Geometry: final body of the model. Coordinates: model frame, mm. Face numbers are marked on the shaded views. A direction names the side the tool comes from. Give positions to 0.01 mm unless a question says otherwise; leave off trailing zeros. Write each loop counter-clockwise with the first axis right and the second up, starting at its lowest first coordinate (ties: lowest second). Pieces come first, ordered by that corner, then holes. Notation, with made-up numbers: M 41,60 L 76,60 A27 ccw 76,91 Z; hole C 33,45.25 d2. An arc over 180 degrees is marked long. Use a Markdown table: item, result. Add a question column.
1) Section A-A on y = 5. Return the cut outline in (x, z), then the cut area to 3 significant figures.
2) Section B-B on x = -9.5. Return the cut outline in (y, z).
3) Set-up query: the marked faces 5, 6 and 7. Return all of +Z, -Z, +X, -X, +Y, -Y with unobstructed straight access to the full face (end or side cutting, diameter ignored); none if empty.
4) Line query: line 1 (Z direction, x = 17.5, y = 14); line 2 (Z direction, x = -27, y = 16); line 3 (Z direction, x = 2, y = 9). Output: solid intervals per line, ascending.
5) Pin query (flat end, axial travel): pin 1 (5 mm diameter, centred on x = 16.5, y = 1, fed in from +Z); pin 2 (1 mm diameter, centred on y = 5, z = 18.5, fed in from +X); pin 3 (1.5 mm diameter, centred on x = 5.5, z = 21, fed in from +Y); pin 4 (8 mm diameter, centred on x = -9.5, y = 12.5, fed in from +Z). Return the tip coordinate at first contact, or that it passes through.
6) Draft query along X for the marked faces 1, 2, 3 and 4. Return one class per face: +X half, -X half, draft (parallel to the pull), parting line (faces both ways), or undercut.
7) Section C-C on y = -6.5. Return the cut outline in (x, z), then the cut area to 3 significant figures.
8) Section D-D on z = 21.5. Return the cut outline in (x, y).
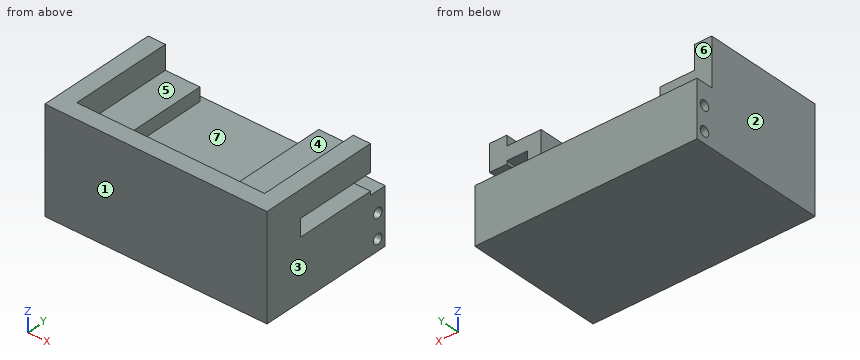
```python
from build123d import *

# Parameters (mm, degrees)
ESQUISSE1_W             = 54.5
ESQUISSE1_H             = 30
BOSS_EXTRU_8_DEPTH      = 5
ESQUISSE7_W             = 30
ESQUISSE7_H             = 30
BOSS_EXTRU_9_DEPTH      = 5
ESQUISSE8_W             = 30
ESQUISSE8_H             = 30
BOSS_EXTRU_10_DEPTH     = 5
ESQUISSE9_W             = 64.5
ESQUISSE9_H             = 30
BOSS_EXTRU_11_DEPTH     = 5
ESQUISSE10_W            = 5
ESQUISSE10_H            = 30
BOSS_EXTRU_12_DEPTH     = 55
ESQUISSE11_W            = 64.5
ESQUISSE11_H            = 16.16204781
BOSS_EXTRU_13_DEPTH     = 5
ESQUISSE13_W            = 3.918976095
ESQUISSE13_H            = 30
BOSS_EXTRU_14_DEPTH     = 10
ESQUISSE16_W            = 3.9189761
ESQUISSE16_H            = 30
BOSS_EXTRU_15_DEPTH     = 10
ESQUISSE17_W            = 3.9189761
ESQUISSE17_H            = 30
BOSS_EXTRU_16_DEPTH     = 4
ESQUISSE20_W            = 5
ESQUISSE20_H            = 23.625106292
ENL_V_MAT_EXTRU_2_DEPTH = 7
ESQUISSE21_R            = 1.45
ENL_V_MAT_EXTRU_3_DEPTH = 7
ENL_V_START             = -7
ESQUISSE22_R            = 1.45
ENL_V_MAT_EXTRU_4_DEPTH = 7


with BuildPart() as part:
    # Esquisse1 → Boss.-Extru.8 (new body)
    with BuildSketch(Plane.XY):
        with Locations((-8.335450003, 5.161172161)):
            Rectangle(ESQUISSE1_W, ESQUISSE1_H)
    extrude(amount=BOSS_EXTRU_8_DEPTH)

    # Esquisse7 → Boss.-Extru.9 (add)
    with BuildSketch(Plane.ZY.offset(35.585450003)):
        with Locations((15, 5.161172161)):
            Rectangle(ESQUISSE7_W, ESQUISSE7_H)
    extrude(amount=BOSS_EXTRU_9_DEPTH)

    # Esquisse8 → Boss.-Extru.10 (add)
    with BuildSketch(Plane(origin=(18.914549997, 0, 0), x_dir=(0, 0, -1), z_dir=(1, 0, 0))):
        with Locations((-15, 5.161172161)):
            Rectangle(ESQUISSE8_W, ESQUISSE8_H)
    extrude(amount=BOSS_EXTRU_10_DEPTH)

    # Esquisse9 → Boss.-Extru.11 (add)
    with BuildSketch(Plane.XZ.offset(9.838827839)):
        with Locations((-8.335450003, 15)):
            Rectangle(ESQUISSE9_W, ESQUISSE9_H)
    extrude(amount=BOSS_EXTRU_11_DEPTH)

    # Esquisse10 → Boss.-Extru.12 (add)
    with BuildSketch(Plane(origin=(-35.585450003, 0, 0), x_dir=(0, 0, -1), z_dir=(1, 0, 0))):
        with Locations((-13.66204781, 5.161172161)):
            Rectangle(ESQUISSE10_W, ESQUISSE10_H)
    extrude(amount=BOSS_EXTRU_12_DEPTH)

    # Esquisse11 → Boss.-Extru.13 (add)
    with BuildSketch(Plane(origin=(0, 20.161172161, 0), x_dir=(1, 0, 0), z_dir=(0, 1, 0))):
        with Locations((-8.335450003, -8.081023905)):
            Rectangle(ESQUISSE11_W, ESQUISSE11_H)
    extrude(amount=BOSS_EXTRU_13_DEPTH)

    # Esquisse13 → Boss.-Extru.14 (add)
    with BuildSketch(Plane(origin=(-35.585450003, 0, 0), x_dir=(0, 0, -1), z_dir=(1, 0, 0))):
        with Locations((-21.121535857, 5.161172161)):
            Rectangle(ESQUISSE13_W, ESQUISSE13_H)
    extrude(amount=BOSS_EXTRU_14_DEPTH)

    # Esquisse16 → Boss.-Extru.15 (add)
    with BuildSketch(Plane.ZY.offset(-18.914549997)):
        with Locations((25.12153586, 5.161172161)):
            Rectangle(ESQUISSE16_W, ESQUISSE16_H)
    extrude(amount=BOSS_EXTRU_15_DEPTH)

    # Esquisse17 → Boss.-Extru.16 (add)
    with BuildSketch(Plane(origin=(0, 0, 23.16204781), x_dir=(-1, 0, 0), z_dir=(0, 0, -1))):
        with Locations((-10.874038047, 5.161172161)):
            Rectangle(ESQUISSE17_W, ESQUISSE17_H)
    extrude(amount=BOSS_EXTRU_16_DEPTH)

    # Esquisse20 → Enlèv. mat.-Extru.2 (cut)
    with BuildSketch(Plane.ZY.offset(-18.914549997)):
        with Locations((19.77668855, 8.348619015)):
            Rectangle(ESQUISSE20_W, ESQUISSE20_H)
    extrude(amount=-ENL_V_MAT_EXTRU_2_DEPTH, mode=Mode.SUBTRACT)

    # Esquisse21 → Enlèv. mat.-Extru.3 (cut)
    with BuildSketch(Plane.ZY.offset(40.585450003)):
        with Locations(Location((3.265574061, 22.632321906, 0), (0, 0, 270))):
            Circle(ESQUISSE21_R)
        with Locations(Location((10.165574061, 22.632321906, 0), (0, 0, 270))):
            Circle(ESQUISSE21_R)
    extrude(amount=-ENL_V_MAT_EXTRU_3_DEPTH, mode=Mode.SUBTRACT)

    # Esquisse22 → Enlèv. mat.-Extru.4 (cut)
    with BuildSketch(Plane(origin=(23.914549997, 0, 0), x_dir=(0, 0, -1), z_dir=(1, 0, 0)).offset(ENL_V_START)):
        with Locations(Location((-3.26557406, 22.632321901, 0), (0, 0, 269.999999963))):
            Circle(ESQUISSE22_R)
        with Locations(Location((-10.16557406, 22.632321901, 0), (0, 0, 269.999999963))):
            Circle(ESQUISSE22_R)
    extrude(amount=ENL_V_MAT_EXTRU_4_DEPTH, mode=Mode.SUBTRACT)


solid = part.part
```
Found:
| question | item | result |
|---|---|---|
| 1 | outline | M -40.59,0 L 23.91,0 L 23.91,17.28 L 18.91,17.28 L 18.91,16.16 L -35.59,16.16 L -35.59,19.16 L -25.59,19.16 L -25.59,23.08 L -35.59,23.08 L -35.59,30 L -40.59,30 Z; M 8.91,19.16 L 12.83,19.16 L 12.83,23.16 L 18.91,23.16 L 18.91,22.28 L 23.91,22.28 L 23.91,30 L 18.91,30 L 18.91,27.08 L 8.91,27.08 Z; hole M -35.59,5 L 18.91,5 L 18.91,11.16 L -35.59,11.16 Z |
| 1 | area | 914 mm² |
| 2 | outline | M -14.84,0 L 25.16,0 L 25.16,16.16 L -9.84,16.16 L -9.84,30 L -14.84,30 Z; hole M -9.84,5 L 20.16,5 L 20.16,11.16 L -9.84,11.16 Z |
| 3 | face 5 | +Z, +Y |
| 3 | face 6 | +Z, +X, -X, +Y |
| 3 | face 7 | +Y |
| 4 | line 1 | 0 to 5, 11.16 to 16.16, 23.16 to 27.08 |
| 4 | line 2 | 0 to 5, 11.16 to 16.16, 19.16 to 23.08 |
| 4 | line 3 | 0 to 5, 11.16 to 16.16 |
| 5 | pin 1 | z = 30 |
| 5 | pin 2 | x = -35.59 |
| 5 | pin 3 | y = -9.84 |
| 5 | pin 4 | z = 16.16 |
| 6 | face 1 | draft |
| 6 | face 2 | -X half |
| 6 | face 3 | +X half |
| 6 | face 4 | undercut |
| 7 | outline | M -40.59,0 L 23.91,0 L 23.91,30 L 18.91,30 L 18.91,27.08 L 8.91,27.08 L 8.91,19.16 L 12.83,19.16 L 12.83,23.16 L 18.91,23.16 L 18.91,16.16 L -35.59,16.16 L -35.59,19.16 L -25.59,19.16 L -25.59,23.08 L -35.59,23.08 L -35.59,30 L -40.59,30 Z; hole M -35.59,5 L 18.91,5 L 18.91,11.16 L -35.59,11.16 Z |
| 7 | area | 939 mm² |
| 8 | outline | M -40.59,-14.84 L 23.91,-14.84 L 23.91,-3.46 L 18.91,-3.46 L 18.91,-9.84 L 12.83,-9.84 L 12.83,20.16 L 8.91,20.16 L 8.91,-9.84 L -25.59,-9.84 L -25.59,20.16 L -40.59,20.16 Z |
